Source: CAD feature listing. Evaluate the final solid. Frame: model axes, mm. Face numbers are marked on the shaded views. A direction names the side the tool comes from. Coordinates: 2 decimals unless noted, no trailing zeros. Order: outer loops, then holes, each group sorted by start corner. A loop starts at its lowest first (then second) coordinate and runs counter-clockwise, first axis right, second up. Notation, with made-up numbers: (0, 31.5) - (34, 31.5) arc R16 cw to (34, 43.5) - close; hole circle Ø8 at (20, 89). An arc over 180 degrees is marked (long way). One line per question, with ' | ' between items.
from build123d import *

# Parameters (mm, degrees)
SKETCH1_R                    = 2
BOSS_EXTRUDE1_DEPTH          = 12
SKETCH2_R                    = 2
SKETCH2_R_2                  = 1
BOSS_EXTRUDE2_DEPTH          = 3
FILLET1_R                    = 10
SKETCH3_W                    = 12
SKETCH3_H                    = 1
CUT_EXTRUDE_THIN2_DEPTH      = 10
CUT_EXTRUDE_THIN2_DEPTH_BACK = 5


with BuildPart() as part:
    # Sketch1 → Boss-Extrude1 (new body)
    with BuildSketch(Plane.XY):
        with BuildLine():
            Line((5, 13.076696831), (5, 45))
            ThreePointArc((5, 45), (0, 50), (-5, 45))
            Line((-5, 45), (-5, 13.076696831))
            ThreePointArc((-5, 13.076696831), (-13.551764697, 3.514210239), (-10.724622204, -8.999026536))
            Line((-10.724622204, -8.999026536), (-8.426488874, -7.070663707))
            ThreePointArc((-8.426488874, -7.070663707), (-3.762221577, 10.336618829), (11, 0))
            ThreePointArc((11, 0), (10.336618829, -3.762221577), (8.426488874, -7.070663707))
            Line((8.426488874, -7.070663707), (10.724622204, -8.999026536))
            ThreePointArc((10.724622204, -8.999026536), (13.551764697, 3.514210239), (5, 13.076696831))
        make_face()
        with BuildLine():
            ThreePointArc((-2, 37.335582027), (0, 39.335582027), (2, 37.335582027))
            Line((2, 37.335582027), (2, 20.741114804))
            ThreePointArc((2, 20.741114804), (0, 18.741114804), (-2, 20.741114804))
            Line((-2, 20.741114804), (-2, 37.335582027))
        make_face(mode=Mode.SUBTRACT)
        with Locations((0, 45)):
            Circle(SKETCH1_R, mode=Mode.SUBTRACT)
    extrude(amount=BOSS_EXTRUDE1_DEPTH)

    # Sketch2 → Boss-Extrude2 (add)
    with BuildSketch(Plane.XY.offset(12)):
        with Locations((0, 45)):
            Circle(SKETCH2_R)
        with Locations((0, 45)):
            Circle(SKETCH2_R_2, mode=Mode.SUBTRACT)
    extrude(amount=-BOSS_EXTRUDE2_DEPTH)

    # Fillet1
    fillet1_edges = [part.edges().sort_by_distance(p)[0] for p in [
        (5, 13.076696831, 6),
        (-5, 13.076696831, 6),
    ]]
    fillet(fillet1_edges, radius=FILLET1_R)

    # Sketch3 → Cut-Extrude-Thin2 (cut, two sides)
    with BuildSketch(Plane(origin=(5, 0, 0), x_dir=(0, 0, -1), z_dir=(1, 0, 0))) as cut_extrude_thin2_sk:
        with Locations((-6, 45)):
            Rectangle(SKETCH3_W, SKETCH3_H)
    extrude(amount=CUT_EXTRUDE_THIN2_DEPTH, mode=Mode.SUBTRACT)
    extrude(cut_extrude_thin2_sk.sketch, amount=-CUT_EXTRUDE_THIN2_DEPTH_BACK, mode=Mode.SUBTRACT)


solid = part.part
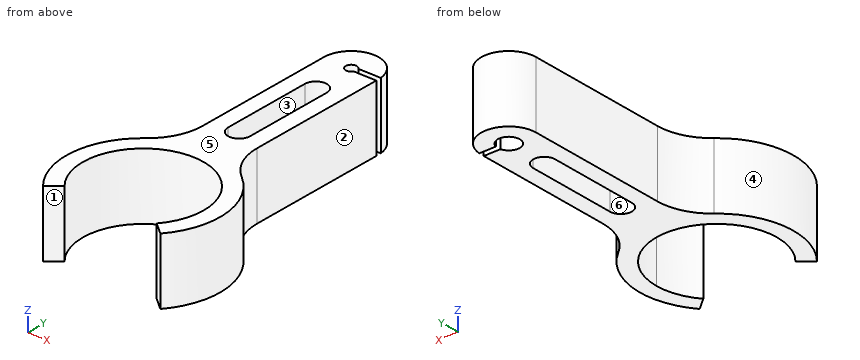
(1) Pin query (flat end, axial travel): P1, Ø2, axis at y = 5, z = 1.5, coming from the -X side; P2, Ø8, axis at x = 0, y = 39, coming from the +Z side; P3, Ø6, axis at y = 25.5, z = 5, coming from the -X side; P4, Ø4, axis at x = 4.5, z = 9.5, coming from the -Y side. Return the tip coordinate at first contact, or that it passes through.
Taken from the geometry:
P1: stops at x = -13.42 | P2: stops at z = 12 | P3: stops at x = -5 | P4: stops at y = 8.87
(2) Pull-direction query (Y, two-part tool) for the marked faces 4, 5 and 6; classes: pulls with the +Y half, pulls with the -Y half, needs draft (parallel to the pull), parting line crosses it, or undercut.
Taken from the geometry:
face 4: parting line crosses it | face 5: needs draft | face 6: undercut
(3) Cut plane C-C (x = 0). Return the cut outline in (y, z), and give its area (3 significant figures).
Taken from the geometry:
outline: (11, 0) - (18.74, 0) - (18.74, 12) - (11, 12) - close; (39.34, 0) - (43, 0) - (43, 9) - (44, 9) - (44, 12) - (39.34, 12) - close; (46, 9) - (47, 9) - (47, 0) - (50, 0) - (50, 12) - (46, 12) - close | area: 179 mm²
(4) Set-up query: the marked faces 1, 2 and 3. Return all of +Z, -Z, +X, -X, +Y, -Y with unobstructed straight access to the full face (end or side cutting, diameter ignored); none if empty.
Taken from the geometry:
face 1: +Z, -Z, -Y | face 2: +Z, -Z, +X, +Y | face 3: +Z, -Z
(5) Cut plane A-A (y = 23). Return the cut outline in (x, z), and give its area (3 significant figures).
Taken from the geometry:
outline: (-5, 0) - (-2, 0) - (-2, 12) - (-5, 12) - close; (2, 0) - (5, 0) - (5, 12) - (2, 12) - close | area: 72.0 mm²
(6) Material intervals for L1, parallel to Y at x = 0, z = 8.25; L2, parallel to Y at x = 1.25, z = 9.5; L3, parallel to X at y = 23.5, z = 2.5, sorted ascending. Write a range as from..to.
Taken from the geometry:
L1: y = 11..18.74, 39.34..43, 47..50 | L2: y = 10.93..19.18, 38.9..44.5, 45.5..49.84 | L3: x = -5..-2, 2..5
(7) Cut plane D-D (x = -3.5). Return the cut outline in (y, z), and give its area (3 significant figures).
Taken from the geometry:
outline: (10.43, 0) - (48.57, 0) - (48.57, 12) - (10.43, 12) - close | area: 458 mm²
